Autodesk Inventor part; units mm, degrees
ref_plane "YZ Plane" through (0, 0, 0) normal (1, 0, 0) x (0, 1, 0)
ref_plane "XZ Plane" through (0, 0, 0) normal (0, 1, 0) x (-1, 0, 0)
ref_plane "XY Plane" through (0, 0, 0) normal (0, 0, 1) x (1, 0, 0)
sketch "Эскиз1" plane through (0, 0, 0) normal (0, 0, 1) x (1, 0, 0)
  line L0 (10, -28.5) -> (-10, -28.5)
  line L1 (-10, -28.5) -> (-10, 28.5)
  line L2 (-10, 28.5) -> (10, 28.5)
  line L3 (10, 28.5) -> (10, -28.5)
  line L4 (10, -28.5) -> (-10, 28.5) construction
  line L5 (-10, -28.5) -> (10, 28.5) construction
  line L6 (-10, 28.5) -> (-27, 28.5)
  line L7 (-27, 28.5) -> (-27, -28.5)
  line L8 (-27, -28.5) -> (-10, -28.5)
  line L9 (-10, -28.5) -> (-10, 28.5)
  line L10 (-27, -28.5) -> (-27, 28.5)
  line L11 (10, 28.5) -> (-10, 28.5)
  line L12 (-10, 28.5) -> (-10, 25.5)
  line L13 (-10, 25.5) -> (10, 25.5)
  line L14 (10, 25.5) -> (10, 28.5)
  line L15 (10, 25.5) -> (7, 25.5)
  line L16 (7, 25.5) -> (7, -28.5)
  line L17 (7, -28.5) -> (10, -28.5)
  line L18 (10, -28.5) -> (10, 25.5)
  line L19 (7, 25.5) -> (-3, 25.5)
  line L20 (-3, 25.5) -> (-3, 28.5)
  line L21 (-3, 28.5) -> (7, 28.5)
  line L22 (7, 28.5) -> (7, 25.5)
  line L23 (-10, 25.5) -> (-3, 28.5)
  line L24 (-3, 25.5) -> (-10, 28.5)
  line L25 (-6.5, 27) -> (-6.5, 17)
  line L26 (7, 25.5) -> (10, 25.5)
  line L27 (10, 25.5) -> (10, 13.5)
  line L28 (10, 13.5) -> (7, 13.5)
  line L29 (7, 13.5) -> (7, 25.5)
  line L30 (7, 25.5) -> (10, 13.5)
  line L31 (7, 13.5) -> (10, 25.5)
  line L32 (8.5, 19.5) -> (0, 19.5)
  line L33 (-6.5, 27) -> (-5.15, 27)
  line L34 (-5.15, 27) -> (-5.15, 28.5)
  line L35 (-5.15, 28.5) -> (-6.5, 28.5)
  line L36 (-6.5, 28.5) -> (-6.5, 27)
  line L37 (-5.15, 28.5) -> (-7.85, 28.5)
  line L38 (-7.85, 28.5) -> (-7.85, 8.5)
  line L39 (-7.85, 8.5) -> (-5.15, 8.5)
  line L40 (-5.15, 8.5) -> (-5.15, 28.5)
  line L41 (-5.15, 25.5) -> (-4.05, 25.5)
  line L42 (-4.05, 25.5) -> (-4.05, 22.5)
  line L43 (-4.05, 22.5) -> (-5.15, 22.5)
  line L44 (-5.15, 22.5) -> (-5.15, 25.5)
  line L45 (-4.05, 22.5) -> (-8.95, 22.5)
  line L46 (-8.95, 22.5) -> (-8.95, 20.6)
  line L47 (-8.95, 20.6) -> (-4.05, 20.6)
  line L48 (-4.05, 20.6) -> (-4.05, 22.5)
  line L49 (8.5, 19.5) -> (10, 19.5)
  line L50 (10, 19.5) -> (10, 18.15)
  line L51 (10, 18.15) -> (8.5, 18.15)
  line L52 (8.5, 18.15) -> (8.5, 19.5)
  line L53 (10, 18.15) -> (0, 18.15)
  line L54 (0, 18.15) -> (0, 20.85)
  line L55 (0, 20.85) -> (10, 20.85)
  line L56 (10, 20.85) -> (10, 18.15)
  line L57 (7, 18.15) -> (4, 18.15)
  line L58 (4, 18.15) -> (4, 17.05)
  line L59 (4, 17.05) -> (7, 17.05)
  line L60 (7, 17.05) -> (7, 18.15)
  line L61 (4, 17.05) -> (2.1, 17.05)
  line L62 (2.1, 17.05) -> (2.1, 21.95)
  line L63 (2.1, 21.95) -> (4, 21.95)
  line L64 (4, 21.95) -> (4, 17.05)
  line L65 (7, 13.5) -> (10, 13.5)
  line L66 (10, 13.5) -> (10, 1.5)
  line L67 (10, 1.5) -> (7, 1.5)
  line L68 (7, 1.5) -> (7, 13.5)
  line L69 (7, 1.5) -> (10, 1.5)
  line L70 (10, 1.5) -> (10, -10.5)
  line L71 (10, -10.5) -> (7, -10.5)
  line L72 (7, -10.5) -> (7, 1.5)
  line L73 (8.5, 7.5) -> (7, 7.5)
  line L74 (10, -3.15) -> (0, -3.15)
  line L75 (0, -5.85) -> (10, -5.85)
  line L76 (4, -2.05) -> (2.1, -2.05)
  line L77 (2.1, -2.05) -> (2.1, -6.95)
  line L78 (2.1, -6.95) -> (4, -6.95)
  line L79 (4, -6.95) -> (4, -2.05)
  line L80 (0, -5.85) -> (-6, -5.85)
  line L81 (-6, -3.15) -> (0, -3.15)
  line L82 (0, -3.15) -> (0, -5.85)
  line L83 (10, -5.85) -> (-10, -5.85)
  line L84 (-10, -5.85) -> (-10, -3.15)
  line L85 (-10, -3.15) -> (10, -3.15)
  line L86 (10, -3.15) -> (10, -5.85)
  line L87 (-27, 28.5) -> (-27, 8)
  line L88 (-17.0714, 4) -> (0.879, 4) construction
  line L89 (-10, -12.4989) -> (10, -12.4989)
  circle A0 centre (-27, 8) radius 3.85
  line L90 (-27, 28.5) -> (-33, 28.5)
  line L91 (-33, 28.5) -> (-33, -28.5)
  line L92 (-33, -28.5) -> (-27, -28.5)
  line L93 (-27, -28.5) -> (-27, 28.5)
  circle A1 centre (-27, 8) radius 6
  line L94 (-10, 28.5) -> (-24.5, 14)
  line L95 (-10, 28.5) -> (10.5061, 28.5) construction
  line L96 (-24.5, 14) -> (-27, 14)
  line L97 (-10, -12.4989) -> (-24.5, 2.0011)
  line L98 (-10, -12.4989) -> (10.5061, -12.4989) construction
  line L99 (-24.5, 2.0011) -> (-27, 2)
  point P0 (0, 0)
  point P1 (2.1, 18.15)
  point P2 (2.1, 20.85)
  point P3 (4, 20.85)
  point P4 (7, 20.85)
  point P5 (7, 28.5)
  point P6 (-3, 25.5)
  point P7 (-5.15, 20.6)
  point P8 (-7.85, 20.6)
  point P9 (-7.85, 22.5)
  point P10 (-7.85, 25.5)
  point P11 (7, -5.85)
  point P12 (4, -5.85)
  point P13 (2.1, -5.85)
  point P14 (2.1, -3.15)
  point P15 (4, -3.15)
  point P16 (7, -3.15)
  point P17 (7, 18.15)
  point P18 (2.1, -5.85)
  point P19 (7, -5.85)
  point P20 (4, -5.85)
  point P21 (-10, -28.5)
  point P22 (-27, 12)
  point P23 (-27, 4)
  point P24 (7, -12.4989)
  dimension "d0" = 20
  dimension "d1" = 57
  dimension "d2" = 17
  dimension "d4" = 3
  dimension "d5" = 3
  dimension "d6" = 10
  dimension "d7" = 10
  dimension "d8" = 12
  dimension "d9" = 1.35
  dimension "d10" = 2.7
  dimension "d11" = 20
  dimension "d12" = 1.1
  dimension "d13" = 3
  dimension "d14" = 4.9
  dimension "d15" = 1.9
  dimension "d16" = 1.35
  dimension "d17" = 2.7
  dimension "d18" = 3
  dimension "d19" = 1.1
  dimension "d20" = 1.9
  dimension "d21" = 4.9
  dimension "d22" = 12
  dimension "d23" = 12
  dimension "d27" = 20
  dimension "d28" = 20.5
  dimension "d31" = 7.7
  dimension "d32" = 6
  dimension "d33" = 135
  dimension "d34" = 135
extrude "Выдавливание1" add sketch "Эскиз1" along normal blind 3 contours L7 A0 A1 | L89 L1 L83 L80 L75 L77 L78 L79 L16 | L97 L99 A1 L96 L94 L1 | L1 L13 L38 L45 L46 L47 L39 L40 L48 L42 L16 L55 L64 L63 L62 L54 L53 L61 L59 L74 L79 L76 L77 L81 L85 | L67 L16 L28 L3 | L59 L58 L53 L16 | L13 L42 L43 L40 | L2 L22 L13 L20
properties part number "крепление оси"
For this review, take the finished solid that the model builds, in its own axes (mm). A direction names the side the tool comes from. Coordinates: 2 decimals unless noted, no trailing zeros. Write each loop counter-clockwise with the first axis right and the second up, starting at its lowest first coordinate (ties: lowest second). Pieces come first, ordered by that corner, then holes. Notation, with made-up numbers: (10, 8.25) -> (37, 8.25) arc R14 ccw to (37, 21.25) -> close; hole circle Ø10 at (-36, 9). An arc over 180 degrees is marked (long way). Put each result on its own line as item: value.
Q1. Take a section at A-A, the plane x = -7. State the section outline as (y, z) points, then the cut area to 3 significant figures.
From the geometry:
outline: (-12.5, 0) -> (-5.85, 0) -> (-5.85, 3) -> (-12.5, 3) -> close; (-3.15, 0) -> (8.5, 0) -> (8.5, 3) -> (-3.15, 3) -> close
area: 54.9 mm2
Q2. Take a section at B-B, the plane y = 8. State the section outline as (x, z) points, then the cut area to 3 significant figures.
From the geometry:
outline: (-33, 0) -> (-30.85, 0) -> (-30.85, 3) -> (-33, 3) -> close; (-23.15, 0) -> (10, 0) -> (10, 3) -> (-23.15, 3) -> close
area: 106 mm2
Q3. Take a section at C-C, the plane y = -10. State the section outline as (x, z) points, then the cut area to 3 significant figures.
From the geometry:
outline: (-12.5, 0) -> (7, 0) -> (7, 3) -> (-12.5, 3) -> close
area: 58.5 mm2
Q4. The part is to be moulded in two halves that separate along Y. For faces 1 (the flat face through (-9, 25.5, 1)), 2 (the flat face through (3, 21.95, 1)), 3 (the flat face through (-17.1, -5.4, 1.5)), say which applies: +Y half, -Y half, draft (parallel to the pull), parting line (faces both ways), or undercut.
From the geometry:
face 1: +Y half
face 2: undercut
face 3: -Y half
Q5. Clearance check with flat-ended pins moving along their axes: pin 1 Ø0.6 at (y, z) = (-6.5, 1) entering from -X; pin 2 Ø5 at (x, y) = (4.5, -5.5) entering from +Z; pin 3 Ø0.9 at (y, z) = (27, 2) entering from -X; pin 4 Ø1.5 at (y, z) = (-1.5, 1) entering from +X. State where each tip first meets the part, or that it passes through.
From the geometry:
pin 1: stops at x = -16.3
pin 2: stops at z = 3
pin 3: stops at x = -11.95
pin 4: stops at x = 7
Q6. Tool access review of faces 4 (the flat face through (1, 18.15, 1)), 5 (the flat face through (-7, 8.5, 1)), 6 (the flat face through (-8, 22.5, 1)), 7 (the flat face through (-17.1, 21.4, 1.5)): name each direction out of +Z, -Z, +X, -X, +Y, -Y from which nothing blocks a thin tool from reaching the whole face with its end or side.
From the geometry:
face 4: +Z, -Z, +X
face 5: +Z, -Z, +Y
face 6: +Z, -Z
face 7: +Z, -Z, -X, +Y
Q7. Wall thickness on L1, parallel to Y at x = -27, z = 1.45; L2, parallel to X at y = 8, z = 0.85; L3, parallel to Y at x = -9, z = 1.65: over which ranges is each line inside the solid? List them lowest first.
From the geometry:
L1: y = 2 to 4.15, 11.85 to 14
L2: x = -33 to -30.85, -23.15 to 10
L3: y = -12.5 to -5.85, -3.15 to 25.5
